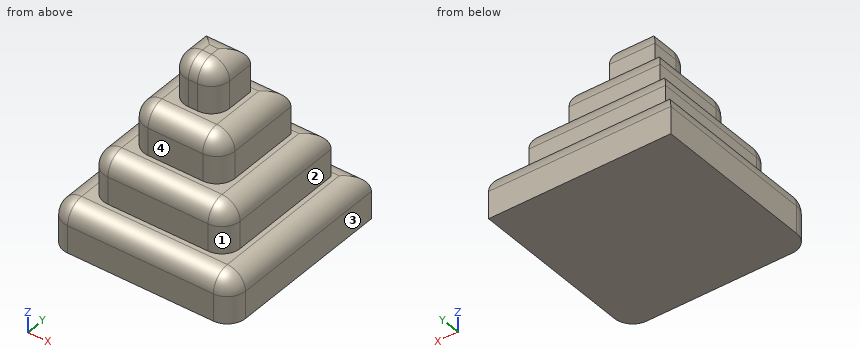
```python
from build123d import *

# Parameters (mm, degrees)
F1_W     = 25
F1_H     = 25
F1_W_2   = 18.75
F1_H_2   = 18.75
F2_DEPTH = 6.25
F1_W_3   = 12.5
F1_H_3   = 12.5
F3_DEPTH = 12.5
F1_W_4   = 6.25
F1_H_4   = 6.25
F4_DEPTH = 18.75
F5_DEPTH = 25
F6_R     = 2.5


with BuildPart() as f2:
    # F1 (on Top) → F2 (new body)
    with BuildSketch(Plane.XY):
        with Locations((12.5, 12.5)):
            Rectangle(F1_W, F1_H)
        with Locations((12.5, 12.5)):
            Rectangle(F1_W_2, F1_H_2, mode=Mode.SUBTRACT)
    extrude(amount=F2_DEPTH)

    # F1 (on Top) → F3 (join)
    with BuildSketch(Plane.XY):
        with Locations((12.5, 12.5)):
            Rectangle(F1_W_2, F1_H_2)
        with Locations((12.5, 12.5)):
            Rectangle(F1_W_3, F1_H_3, mode=Mode.SUBTRACT)
    extrude(amount=F3_DEPTH)

    # F1 (on Top) → F4 (join)
    with BuildSketch(Plane.XY):
        with Locations((12.5, 12.5)):
            Rectangle(F1_W_3, F1_H_3)
        with Locations((12.5, 12.5)):
            Rectangle(F1_W_4, F1_H_4, mode=Mode.SUBTRACT)
    extrude(amount=F4_DEPTH)

    # F1 (on Top) → F5 (join)
    with BuildSketch(Plane.XY):
        with Locations((12.5, 12.5)):
            Rectangle(F1_W_4, F1_H_4)
    extrude(amount=F5_DEPTH)

    # F6
    f6_edges = [f2.edges().sort_by_distance(p)[0] for p in [
        (18.75, 12.5, 18.75),
        (12.5, 18.75, 18.75),
        (6.25, 12.5, 18.75),
        (12.5, 6.25, 18.75),
        (12.5, 15.625, 25),
        (9.375, 12.5, 25),
        (12.5, 9.375, 25),
        (15.625, 12.5, 25),
        (12.5, 3.125, 12.5),
        (21.875, 12.5, 12.5),
        (12.5, 21.875, 12.5),
        (3.125, 12.5, 12.5),
        (12.5, 25, 6.25),
        (0, 12.5, 6.25),
        (12.5, 0, 6.25),
        (15.625, 9.375, 21.875),
        (9.375, 9.375, 21.875),
        (6.25, 6.25, 15.625),
        (18.75, 6.25, 15.625),
        (3.125, 3.125, 9.375),
        (21.875, 3.125, 9.375),
        (25, 12.5, 6.25),
        (25, 0, 3.125),
        (0, 0, 3.125),
    ]]
    fillet(f6_edges, radius=F6_R)


solid = f2.part
```
Input: part model. Units: mm. Frame: model coordinates. Face numbers are marked on the shaded views. A direction names the side the tool comes from. Give positions to 0.01 mm unless a question says otherwise; leave off trailing zeros. Order: outer loops, then holes, each group sorted by start corner. A loop starts at its lowest first (then second) coordinate and runs counter-clockwise, first axis right, second up.
1. Section D-D on x = 18.25. Return the cut outline in (y, z) (3 decimals), and give its area (3 significant figures).
Derived:
outline: (0, 0) - (25, 0) - (25, 3.75) arc R2.5 ccw to (22.5, 6.25) - (21.875, 6.25) - (21.875, 10) arc R2.5 ccw to (19.375, 12.5) - (18.75, 12.5) - (18.75, 16.25) arc R2.5 ccw to (18.25, 17.75) - (8.75, 17.75) arc R1.5 ccw to (7.25, 16.25) - (7.25, 12.5) - (5.625, 12.5) arc R2.5 ccw to (3.125, 10) - (3.125, 6.25) - (2.5, 6.25) arc R2.5 ccw to (0, 3.75) - close
area: 328 mm2
2. Reachability of the marked faces 1, 2, 3 and 4 from +Z, -Z, +X, -X, +Y, -Y: full face, straight path, thin tool, end or side. Return the list, or none.
Derived:
face 1: +Z, +X, -Y
face 2: +Z, +X, +Y, -Y
face 3: +Z, -Z, +X, +Y, -Y
face 4: +Z, +X, -X, -Y
3. Pin query (flat end, axial travel): pin 1 (3 mm diameter, centred on y = 12.5, z = 14.5, fed in from +X); pin 2 (3 mm diameter, centred on x = 11, z = 8, fed in from -Y) (3 decimals); pin 3 (1.1 mm diameter, centred on x = 10, z = 8, fed in from +Y) (3 decimals). Return the tip coordinate at first contact, or that it passes through.
Derived:
pin 1: stops at x = 18.75
pin 2: stops at y = 3.125
pin 3: stops at y = 21.875
4. Section B-B on z = 7.5. Return the cut outline in (x, y) (3 decimals).
Derived:
outline: (3.125, 5.625) arc R2.5 ccw to (5.625, 3.125) - (19.375, 3.125) arc R2.5 ccw to (21.875, 5.625) - (21.875, 21.875) - (3.125, 21.875) - close
5. Section A-A on x = 12.5. Return the cut outline in (y, z) (3 decimals).
Derived:
outline: (0, 0) - (25, 0) - (25, 3.75) arc R2.5 ccw to (22.5, 6.25) - (21.875, 6.25) - (21.875, 10) arc R2.5 ccw to (19.375, 12.5) - (18.75, 12.5) - (18.75, 16.25) arc R2.5 ccw to (16.25, 18.75) - (15.625, 18.75) - (15.625, 22.5) arc R2.5 ccw to (13.125, 25) - (11.875, 25) arc R2.5 ccw to (9.375, 22.5) - (9.375, 18.75) - (8.75, 18.75) arc R2.5 ccw to (6.25, 16.25) - (6.25, 12.5) - (5.625, 12.5) arc R2.5 ccw to (3.125, 10) - (3.125, 6.25) - (2.5, 6.25) arc R2.5 ccw to (0, 3.75) - close
6. Section C-C on y = 4.75. Return the cut outline in (x, z) (3 decimals).
Derived:
outline: (0, 0) - (25, 0) - (25, 3.75) arc R2.5 ccw to (22.5, 6.25) - (21.717, 6.25) - (21.717, 10) arc R2.342 ccw to (19.375, 12.342) - (5.625, 12.342) arc R2.342 ccw to (3.283, 10) - (3.283, 6.25) - (2.5, 6.25) arc R2.5 ccw to (0, 3.75) - close
7. Material intervals for L1, parallel to Z at x = 19.25, y = 14.5; L2, parallel to X at y = 12.5, z = 14.75; L3, parallel to Z at x = 6, y = 22, sorted ascending.
Derived:
L1: z = 0 to 12.5
L2: x = 6.25 to 18.75
L3: z = 0 to 6.25
